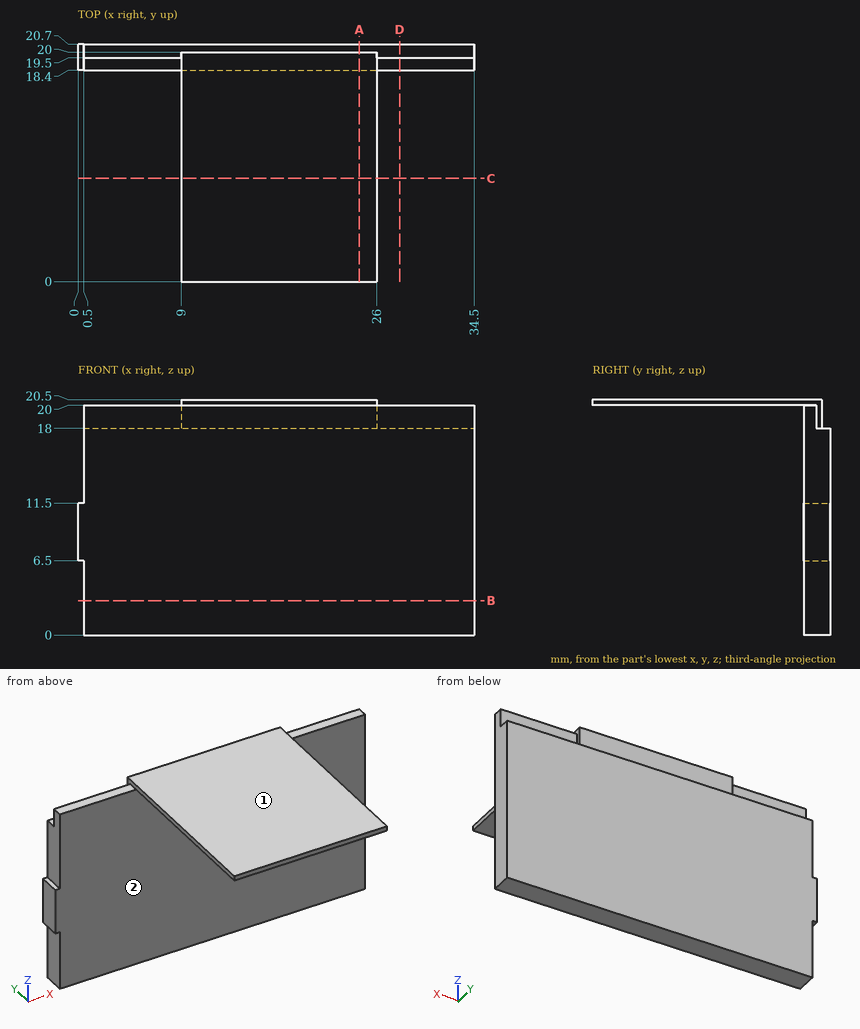
Geometry: see drawing. Coordinates: mm, zero at the bounding-box minimum. A direction names the side the tool comes from. Coordinates: 2 decimals unless noted, no trailing zeros. Write each loop counter-clockwise with the first axis right and the second up, starting at its lowest first coordinate (ties: lowest second). Pieces come first, ordered by that corner, then holes. Notation, with made-up numbers: M 73,7.5 L 85,7.5 A23 ccw 85,21.5 Z; hole C -21.75,-8 d8. An arc over 180 degrees is marked long. Use CSV: the item, a comma, the result in double quotes. Start each with the question number.
1. Cut plane A-A on x = 24.5. Return the cut outline in (y, z), plus the area to 3 significant figures.
2. Ray query, probe 1 along Y at (x, z) = (21, 5.5); probe 2 along Z at (x, y) = (11, 11.25); probe 3 along Y at (x, z) = (23, 19.25). Return the intervals inside material, ascending.
3. Cut plane D-D on x = 28. Return the cut outline in (y, z).
4. Reachability of the marked faces 1 and 2 from +Z, -Z, +X, -X, +Y, -Y: full face, straight path, thin tool, end or side. Return the list, or none.
5. Cut plane B-B on z = 3. Return the cut outline in (x, y), plus the area to 3 significant figures.
6. First-contact query: P1, Ø2, axis at x = 19, z = 7.5, coming from the -Y side; P2, Ø2, axis at x = 18.5, z = 19.5, coming from the +Y side; P3, Ø2.5, axis at y = 19.5, z = 3.5, coming from the -X side. Flat tips, straight axial feed; report the tip coordinate or a pass-through.
7. Cut plane C-C on y = 9. Return the cut outline in (x, z), plus the area to 3 significant figures.
Entries:
1,outline,"M 0,20 L 18.4,20 L 18.4,0 L 20.7,0 L 20.7,18 L 20,18 L 20,20.5 L 0,20.5 Z"
1,area,"54.6 mm²"
2,probe 1,"18.4 to 20.7"
2,probe 2,"20 to 20.5"
2,probe 3,"18.4 to 20"
3,outline,"M 18.4,0 L 20.7,0 L 20.7,18 L 19.5,18 L 19.5,20 L 18.4,20 Z"
4,face 1,"+Z, +X, -X, +Y, -Y"
4,face 2,"-Z, +X, -X, -Y"
5,outline,"M 0.5,18.4 L 34.5,18.4 L 34.5,20.7 L 0.5,20.7 Z"
5,area,"78.2 mm²"
6,P1,"y = 18.4"
6,P2,"y = 20"
6,P3,"x = 0.5"
7,outline,"M 9,20 L 26,20 L 26,20.5 L 9,20.5 Z"
7,area,"8.50 mm²"
